```python
from build123d import *

# Parameters (mm, degrees)
ESQUISSE1_R             = 14
BOSS_EXTRU_1_DEPTH      = 4.5
CONG_1_R                = 2
ESQUISSE14_W            = 2
ESQUISSE14_H            = 2
ESQUISSE15_R            = 7.5
ENL_V_MAT_EXTRU_2_DEPTH = 10


with BuildPart() as part:
    # Esquisse1 → Boss.-Extru.1 (new body, symmetric)
    with BuildSketch(Plane.XY):
        Circle(ESQUISSE1_R)
    extrude(amount=BOSS_EXTRU_1_DEPTH, both=True)

    # Congé1
    cong_1_edges = [part.edges().sort_by_distance(p)[0] for p in [
        (-14, 0, -4.5),
        (-14, 0, 4.5),
    ]]
    fillet(cong_1_edges, radius=CONG_1_R)

    # Esquisse14 → Enlèvement de matière-Révolution2 (revolve, cut)
    with BuildSketch(Plane(origin=(0, 0, 0), x_dir=(0, 0, -1), z_dir=(1, 0, 0))):
        with Locations((0, 13)):
            Rectangle(ESQUISSE14_W, ESQUISSE14_H)
    revolve(axis=Axis((0, 0, 11.517879347), (0, 0, -1)), mode=Mode.SUBTRACT)

    # Esquisse15 → Enlèv. mat.-Extru.2 (cut, through all)
    with BuildSketch(Plane.XY.offset(4.5)):
        Circle(ESQUISSE15_R)
    extrude(amount=-ENL_V_MAT_EXTRU_2_DEPTH, mode=Mode.SUBTRACT)


solid = part.part
```
Could you check a few things on this model? Use its own coordinates, in mm. A direction names the side the tool comes from. Give positions to 0.01 mm unless a question says otherwise; leave off trailing zeros. Loops run counter-clockwise (first coordinate to the right, second up) from the corner with the lowest first, then second, coordinate; pieces in that order, holes last. Notation, with made-up numbers: (34, 26) - (73, 26) arc R24 cw to (73, 64) - close; hole circle Ø3 at (71.25, 19.5). An arc over 180 degrees is marked (long way). Use one line per item in the form item = value.
1. I'm going to push flat-ended pins straight in: pin 1 Ø1.5 at (y, z) = (3, 1) entering from +X; pin 2 Ø1 at (x, z) = (-9, 1.5) entering from -Y; pin 3 Ø5 at (y, z) = (-7.5, -1.5) entering from +X. Where does each tip first touch, or does it pass through?
Response values:
pin_1 = 13.82
pin_2 = -11.12
pin_3 = 13.08
2. On a 3-axis mill with a long thin cutter (end or side, diameter ignored), from which of +Z, -Z, +X, -X, +Y, -Y can I reach the whole of each face in a straight line? I mean faces 1 (the face through (10.4, 6.3, 1)), 2 (the face through (-6, -5, -4.5)). Say none if no direction works.
Response values:
face_1 = none
face_2 = -Z, +X, -X, +Y, -Y
3. I want a section at C-C (z = 0.5). Please give me the cut outline in (x, y).
Response values:
outline = circle Ø24 at (0, 0); hole circle Ø15 at (0, 0)
4. Thinking about a two-plate mould opening in X: for faces 3 (the face through (-6, -5, 4.5)), 4 (the face through (0.53, -11.99, -0.01)), 5 (the face through (-7.493, 0.33, 0.063)), which applies, released by +X, released by -X, zero draft, split by the parting line, or undercut?
Response values:
face_3 = zero draft
face_4 = split by the parting line
face_5 = undercut
5. I need wall thicknesses on probe 1 along Y at (x, z) = (0, -2); probe 2 along X at (y, z) = (-6.25, -0.25); probe 3 along Y at (x, z) = (1, 3.75). Which ranges of each line are inside material? Lowest first, please.
Response values:
probe_1 = -14 to -7.5, 7.5 to 14
probe_2 = -10.24 to -4.15, 4.15 to 10.24
probe_3 = -13.52 to -7.43, 7.43 to 13.52
6. I want a section at A-A (y = 0). Please give me the cut outline in (x, z), and give its area (3 significant figures).
Response values:
outline = (-14, -2.5) arc R2 ccw to (-12, -4.5) - (-7.5, -4.5) - (-7.5, 4.5) - (-12, 4.5) arc R2 ccw to (-14, 2.5) - (-14, 1) - (-12, 1) - (-12, -1) - (-14, -1) - close; (7.5, -4.5) - (12, -4.5) arc R2 ccw to (14, -2.5) - (14, -1) - (12, -1) - (12, 1) - (14, 1) - (14, 2.5) arc R2 ccw to (12, 4.5) - (7.5, 4.5) - close
area = 106 mm²
